Geometry check sheet. Reference: the model listing, model coordinates, mm. Face numbers are marked on the shaded views. A direction names the side the tool comes from. Round coordinates to 2 decimals unless told otherwise and drop trailing zeros. Loops run counter-clockwise (first coordinate to the right, second up) from the corner with the lowest first, then second, coordinate; pieces in that order, holes last. Notation, with made-up numbers: (37.5, 1) -> (64.5, 1) arc R20 cw to (64.5, 15) -> close; hole circle Ø9 at (26, 68.25). An arc over 180 degrees is marked (long way). Use a Markdown table: item, result. Add a question column.
Q1. Sectioned sample at A-A, the plane x = 0. Enter the section's corners in (y, z) (3 decimals).
Q2. Sectioned sample at C-C, the plane y = 0. Enter the section's corners in (x, z) (3 decimals), then the cut area to 4 significant figures.
Q3. Release check for a two-part mould opening along Y. For the marked faces 4, 5 and 6 record: released by +Y, released by -Y, zero draft, split by the parting line, or undercut.
Q4. Sectioned sample at B-B, the plane z = 4. Enter the section's corners in (x, y) (3 decimals).
Q5. Set-up check for the marked faces 1, 2 and 3: record each of +Z, -Z, +X, -X, +Y, -Y from which the full face is reachable in a straight line by a thin tool's end or side.
Q6. Sectioned sample at D-D, the plane y = 12. Enter the section's corners in (x, z), then the cut area to 3 significant figures.
Q7. Gauge pin test, flat ends, axial feed: P1, Ø10, axis at y = 0.5, z = -3, coming from the -X side; P2, Ø10, axis at x = 7, z = -14.5, coming from the +Y side; P3, Ø12, axis at y = -2, z = -2.5, coming from the +X side; P4, Ø2, axis at x = -12, y = -3, coming from the -Z side. Record the tip position at first contact, or that the pin passes through.
Q8. Material ranges on L1, parallel to Y at x = 0, z = -17.5 (3 decimals); L2, parallel to X at y = 7.25, z = -16.5; L3, parallel to Y at x = 0, z = 3 (3 decimals), recorded low to high.
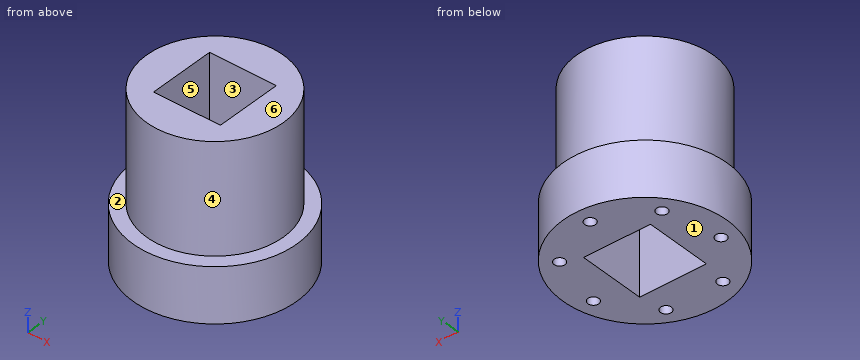
```python
from build123d import *

# Parameters (mm, degrees)
SKETCH1_R           = 12.5
BOSS_EXTRUDE1_DEPTH = 10
SKETCH11_R          = 15
BOSS_EXTRUDE2_DEPTH = 10
SKETCH8_W           = 12.25
SKETCH8_H           = 12.25
CUT_EXTRUDE1_DEPTH  = 37.742346142
SKETCH12_R          = 1
CUT_EXTRUDE2_DEPTH  = 5
CIRPATTERN1_COUNT   = 7


with BuildPart() as part:
    # Sketch1 → Boss-Extrude1 (new, symmetric)
    with BuildSketch(Plane.XY):
        Circle(SKETCH1_R)
    extrude(amount=BOSS_EXTRUDE1_DEPTH, both=True)

    # Sketch11 → Boss-Extrude2 (add)
    with BuildSketch(Plane(origin=(0, 0, -10), x_dir=(-1, 0, 0), z_dir=(0, 0, -1))):
        Circle(SKETCH11_R)
    extrude(amount=BOSS_EXTRUDE2_DEPTH)

    # Sketch8 → Cut-Extrude1 (cut, through all)
    with BuildSketch(Plane.XY.offset(10)):
        Rectangle(SKETCH8_W, SKETCH8_H)
    extrude(amount=-CUT_EXTRUDE1_DEPTH, mode=Mode.SUBTRACT)

    # Sketch12 → Cut-Extrude2 (cut)
    with BuildSketch(Plane(origin=(0, 0, -20), x_dir=(-1, 0, 0), z_dir=(0, 0, -1))):
        with Locations((0, 12.00000002)):
            Circle(SKETCH12_R)
    cut_extrude2 = extrude(amount=-CUT_EXTRUDE2_DEPTH, mode=Mode.SUBTRACT)

    # CirPattern1: Cut-Extrude2 ×7 about axis
    cirpattern1_axis = Axis((0, 0, 0), (0, 0, 1))
    for i in range(1, CIRPATTERN1_COUNT):
        add(cut_extrude2.rotate(cirpattern1_axis, i * 360 / CIRPATTERN1_COUNT), mode=Mode.SUBTRACT)


solid = part.part
```
Values:
| question | item | result |
|---|---|---|
| 1 | outline | (-15, -20) -> (-6.125, -20) -> (-6.125, 10) -> (-12.5, 10) -> (-12.5, -10) -> (-15, -10) -> close; (6.125, -20) -> (11, -20) -> (11, -15) -> (13, -15) -> (13, -20) -> (15, -20) -> (15, -10) -> (12.5, -10) -> (12.5, 10) -> (6.125, 10) -> close |
| 2 | outline | (-15, -20) -> (-6.125, -20) -> (-6.125, 10) -> (-12.5, 10) -> (-12.5, -10) -> (-15, -10) -> close; (6.125, -20) -> (15, -20) -> (15, -10) -> (12.5, -10) -> (12.5, 10) -> (6.125, 10) -> close |
| 2 | area | 432.5 mm^2 |
| 3 | face 4 | split by the parting line |
| 3 | face 5 | undercut |
| 3 | face 6 | zero draft |
| 4 | outline | circle Ø25 at (0, 0); hole (-6.125, -6.125) -> (6.125, -6.125) -> (6.125, 6.125) -> (-6.125, 6.125) -> close |
| 5 | face 1 | -Z, +X, -X, +Y, -Y |
| 5 | face 2 | +Z |
| 5 | face 3 | +Z, -Z |
| 6 | outline | (-9, -20) -> (-1, -20) -> (-1, -15) -> (1, -15) -> (1, -20) -> (9, -20) -> (9, -10) -> (3.5, -10) -> (3.5, 10) -> (-3.5, 10) -> (-3.5, -10) -> (-9, -10) -> close |
| 6 | area | 310 mm^2 |
| 7 | P1 | x = -12.5 |
| 7 | P2 | y = 14.87 |
| 7 | P3 | x = 12.5 |
| 7 | P4 | z = -20 |
| 8 | L1 | -15 to -6.125, 6.125 to 11, 13 to 15 |
| 8 | L2 | -13.13 to -10.35, -8.41 to 8.41, 10.35 to 13.13 |
| 8 | L3 | -12.5 to -6.125, 6.125 to 12.5 |
